Autodesk Inventor part; units mm, degrees
ref_plane "YZ Plane" through (0, 0, 0) normal (1, 0, 0) x (0, 1, 0)
ref_plane "XZ Plane" through (0, 0, 0) normal (0, 1, 0) x (-1, 0, 0)
ref_plane "XY Plane" through (0, 0, 0) normal (0, 0, 1) x (1, 0, 0)
sketch "Sketch1" plane through (0, 0, 0) normal (0, 1, 0) x (-1, 0, 0)
  circle A0 centre (0, 0) radius 16.5
  circle A1 centre (0, 0) radius 14.75
  dimension "d0" = 33
  dimension "d1" = 29.5
extrude "Extrusion1" add sketch "Sketch1" along normal blind 25.4
sketch "Sketch2" plane through (0, 25.4, 0) normal (0, 1, 0) x (1, 0, 0)
  circle A0 centre (0, 0) radius 14.75
  circle A1 centre (0, 0) radius 31.75
  circle A2 centre (0, 0) radius 14.75
  dimension "d5" = 63.5
  dimension "d6" = 0
extrude "Extrusion2" add sketch "Sketch2" along normal blind 2
sketch "Sketch3" plane through (0, 25.4, 0) normal (0, -1, 0) x (1, 0, 0)
  circle A0 centre (0, -20.32) radius 5
  circle A1 centre (0, -21.32) radius 5
  line L0 (0, -20.32) -> (0, -21.32)
  line L1 (5, -20.32) -> (5, -21.32)
  line L2 (-5, -20.32) -> (-5, -21.32)
  point P0 (0, 0)
  point P1 (4.9749, -20.82)
  point P2 (-4.9749, -20.82)
  dimension "d9" = 10
  dimension "d10" = 1
  dimension "d11" = 20.32
extrude "Extrusion3" cut sketch "Sketch3" against normal blind 2 contours A0 A1 | A1 A0 | A0 A1
properties part number "O-Ring"
Part model, mm, in its own coordinate system. A direction names the side the tool comes from. Round coordinates to 2 decimals unless told otherwise and drop trailing zeros. Loops run counter-clockwise (first coordinate to the right, second up) from the corner with the lowest first, then second, coordinate; pieces in that order, holes last.
Item 1: Cut at D-D, the plane z = -4. Give the cut face in (x, y), then the cut area to 3 significant figures.
Item 2: Cut at A-A, the plane z = -24.5. Give the cut face in (x, y).
Item 3: Cut at B-B, the plane y = 3.5. Give the cut face in (x, z).
Item 4: Drop flat-ended pins along their axis: P1, Ø0.6, axis at x = 0.5, z = -16, coming from the +Y side; P2, Ø2, axis at x = -9.5, y = 24.5, coming from the -Z side; P3, Ø12, axis at x = -13, y = 22, coming from the +Z side. Give the stop position or say it passes through.
Item 5: Drill centre lines: line 1 (Z direction, x = 0, y = 26.15); line 2 (X direction, y = 14.75, z = 0); line 3 (Y direction, x = -25, z = -13.5). Where is each one in solid material? Low to high.
Item 6: 3-axis set-ups, long thin cutter, end or side, ignore diameter. For faces 1 (the face through (0.12, 26.39, -15.32)), 2 (the face through (-6.883, 26.386, -30.995)), 3 (the face through (-15.24, 12.52, 6.32)): which of +Z, -Z, +X, -X, +Y, -Y reach the whole face in a straight line?
A:
1. outline: (-31.5, 25.4) - (-16.01, 25.4) - (-16.01, 0) - (-14.2, 0) - (-14.2, 27.4) - (-31.5, 27.4) - close; (14.2, 0) - (16.01, 0) - (16.01, 25.4) - (31.5, 25.4) - (31.5, 27.4) - (14.2, 27.4) - close
1. area: 161 mm2
2. outline: (-20.19, 25.4) - (-3.86, 25.4) - (-3.86, 27.4) - (-20.19, 27.4) - close; (3.86, 25.4) - (20.19, 25.4) - (20.19, 27.4) - (3.86, 27.4) - close
3. outline: circle Ø33 at (0, 0); hole circle Ø29.5 at (0, 0)
4. P1: stops at y = 25.4
4. P2: stops at z = -30.43
4. P3: stops at z = 30.71
5. line 1: z = -31.75 to -26.32, -15.32 to -14.75, 14.75 to 31.75
5. line 2: x = -16.5 to -14.75, 14.75 to 16.5
5. line 3: y = 25.4 to 27.4
6. face 1: +Y
6. face 2: +Y, -Y
6. face 3: -Y
